Build history of the part. All positions in model axes, mm. A direction names the side the tool comes from. Round coordinates to 2 decimals unless told otherwise and drop trailing zeros. Loops run counter-clockwise (first coordinate to the right, second up) from the corner with the lowest first, then second, coordinate; pieces in that order, holes last. Notation, with made-up numbers: (-37, -23) -> (-14, -23) arc R14 cw to (-14, 3) -> close; hole circle Ø3 at (-30.75, -32.75). An arc over 180 degrees is marked (long way). Put each result on its own line as item: value. Start each with the question number.
Autodesk Fusion 360 part; units mm, degrees
sketch "Sketch1" plane through (0, 0, 0) normal (0, 0, 1) x (1, 0, 0)
  line L0 (-50, 0) -> (-15, 0)
  line L1 (-15, 0) -> (-15, 10)
  line L2 (-15, 10) -> (-50, 10)
  line L3 (-50, 10) -> (-50, 0)
  dimension "d1" = 35
  dimension "d2" = 10
extrude "Extrude1" add sketch "Sketch1" along normal blind 10
sketch "Sketch2" plane through (0, 0, 10) normal (0, 0, 1) x (-1, 0, 0)
  line L0 (50, -10) -> (50, 0)
  line L1 (50, 0) -> (15, 0)
  line L2 (15, 0) -> (15, -10)
  line L3 (15, -10) -> (50, -10)
  line L4 (50, -10) -> (50, -5)
  line L5 (15, -5) -> (15, -10)
  line L6 (15, -5) -> (20, -5)
  line L7 (20, -5) -> (50, -5)
  line L8 (50, -10) -> (15, -10)
extrude "Extrude2" add sketch "Sketch2" along normal blind 25 contours L0 L2 L3 L4 L5 L6 L7 L8
sketch "Sketch3" plane through (0, 5, 0) normal (0, -1, 0) x (1, 0, 0)
  line L0 (-50, 10) -> (-15, 10)
  line L1 (-15, 10) -> (-15, 35)
  line L2 (-15, 35) -> (-50, 35)
  line L3 (-50, 35) -> (-50, 10)
  line L4 (-15, 10) -> (-17, 10)
  line L5 (-17, 10) -> (-17, 12)
  circle A0 centre (-17, 12) radius 1.5
  line L6 (-50, 10) -> (-48, 10)
  circle A1 centre (-48, 12) radius 1.5
  dimension "d7" = 2
  dimension "d8" = 2
  dimension "d9" = 3
  dimension "d10" = 2
  dimension "d11" = 3
extrude "Extrude3" cut sketch "Sketch3" against normal blind 15 contours A0 | A1
sketch "Sketch4" plane through (0, 5, 0) normal (0, -1, 0) x (1, 0, 0)
  circle A0 centre (-17, 12) radius 1.5
  circle A1 centre (-48, 12) radius 1.5
  line L0 (-50, 10) -> (-15, 10)
  line L1 (-15, 10) -> (-15, 35)
  line L2 (-15, 35) -> (-50, 35)
  line L3 (-50, 35) -> (-50, 10)
  line L4 (-17, 10) -> (-17, 25)
  line L5 (-48, 10) -> (-48, 25)
  circle A2 centre (-48, 25) radius 1.5
  circle A3 centre (-17, 25) radius 1.5
  dimension "d14" = 15
  dimension "d15" = 15
  dimension "d16" = 3
  dimension "d17" = 3
extrude "Extrude4" cut sketch "Sketch4" against normal blind 24 contours A2 | A3
sketch "Sketch5" plane through (0, 0, 0) normal (0, 0, -1) x (1, 0, 0)
  line L0 (-50, 0) -> (-50, -10)
  line L1 (-50, -10) -> (-15, -10)
  line L2 (-15, -10) -> (-15, 0)
  line L3 (-15, 0) -> (-50, 0)
sketch "Sketch6" plane through (-50, 0, 0) normal (-1, 0, 0) x (0, -1, 0)
  line L0 (-10, 0) -> (0, 0)
  line L1 (0, 0) -> (0, 10)
  line L2 (0, 10) -> (-5, 10)
  line L3 (-5, 10) -> (-5, 35)
  line L4 (-5, 35) -> (-10, 35)
  line L5 (-10, 35) -> (-10, 0)
  line L6 (0, 10) -> (-10, 10)
  line L7 (-10, 10) -> (-10, 0)
  line L8 (-10, 0) -> (0, 0)
  line L9 (0, 0) -> (0, 10)
extrude "Extrude5" add sketch "Sketch6" along normal blind 3 contours L0 L1 L2 L5 L6 L7 L8 L9
sketch "Sketch7" plane through (-15, 0, 0) normal (1, 0, 0) x (0, 1, 0)
  line L0 (0, 0) -> (10, 0)
  line L1 (10, 0) -> (10, 35)
  line L2 (10, 35) -> (5, 35)
  line L3 (5, 35) -> (5, 10)
  line L4 (5, 10) -> (0, 10)
  line L5 (0, 10) -> (0, 0)
  line L6 (0, 10) -> (10, 10)
  line L7 (10, 10) -> (10, 0)
  line L8 (10, 0) -> (0, 0)
  line L9 (0, 0) -> (0, 10)
extrude "Extrude6" add sketch "Sketch7" along normal blind 3 contours L0 L1 L4 L5 L6 L7 L8 L9
sketch "Sketch8" plane through (0, 0, 0) normal (0, 0, -1) x (1, 0, 0)
sketch "Sketch9" plane through (0, 0, 0) normal (0, 0, -1) x (1, 0, 0)
  line L0 (-53, -10) -> (-52, -10)
  line L1 (-52, -10) -> (-32, -10)
  line L2 (-32, -10) -> (-32, -5)
  line L3 (-32, -5) -> (-15, -5)
  line L4 (-32, -5) -> (-49, -5)
  line L5 (-49, -5) -> (-49, -1)
  line L6 (-49, -5) -> (-49, -9)
  line L7 (-49, -1) -> (-15, -1)
  line L8 (-15, -1) -> (-15, -9)
  line L9 (-15, -9) -> (-49, -9)
  dimension "d24" = 20
  dimension "d25" = 17
  dimension "d26" = 17
  dimension "d27" = 4
  dimension "d28" = 4
extrude "Extrude7" cut sketch "Sketch9" against normal blind 5
Item 1: Cut at D-D on z = 3. Write the cut outline in (x, y).
Item 2: Drop flat-ended pins along their axis: pin 1 (4 mm diameter, centred on y = 8, z = 24, fed in from -X); pin 2 (2.5 mm diameter, centred on x = -33, y = 5.5, fed in from -Z); pin 3 (4 mm diameter, centred on y = 8, z = 21, fed in from +X). Give the stop position or say it passes through.
Item 3: Cut at C-C on y = 8.5. Write the cut outline in (x, z).
Item 4: Cut at B-B on z = 25. Write the cut outline in (x, y), then the cut area to 3 significant figures.
Item 5: Pull direction Z, two halves, no side cores. Call faces 1 (the face through (-49.11, 7.46, 26.01)), 2 (the face through (-49, 5, 2)), 3 (the face through (-32.8, 0.5, 0)): +Z half, -Z half, draft (parallel to the pull), parting line (faces both ways), or undercut.
Item 6: Wall check: line 1 (Z direction, x = -48, y = 6); line 2 (X direction, y = 7, z = 25); line 3 (Y direction, x = -45, z = 3). Give the ranges that are in metal, low to high. Write a range as from..to.
Item 7: 3-axis set-ups, long thin cutter, end or side, ignore diameter. For faces 4 (the face through (-50, 8, 22)), 5 (the face through (-32, 5, 22)), 6 (the face through (-15, 7, 22)), 7 (the face through (-33, 10, 17)), 8 (the face through (-32, 9, 2)): which of +Z, -Z, +X, -X, +Y, -Y reach the whole face in a straight line?
Item 8: Cut at A-A on x = -48. Write the cut outline in (y, z), then the cut area to 3 significant figures.
Ans:
1. outline: (-53, 0) -> (-12, 0) -> (-12, 10) -> (-53, 10) -> close; hole (-49, 1) -> (-15, 1) -> (-15, 9) -> (-49, 9) -> close
2. pin 1: stops at x = -50
2. pin 2: stops at z = 5
2. pin 3: stops at x = -15
3. outline: (-53, 0) -> (-49, 0) -> (-49, 5) -> (-15, 5) -> (-15, 0) -> (-12, 0) -> (-12, 10) -> (-15, 10) -> (-15, 35) -> (-50, 35) -> (-50, 10) -> (-53, 10) -> close; hole circle Ø3 at (-48, 12); hole circle Ø3 at (-48, 25); hole circle Ø3 at (-17, 12); hole circle Ø3 at (-17, 25)
4. outline: (-50, 5) -> (-49.5, 5) -> (-49.5, 10) -> (-50, 10) -> close; (-46.5, 5) -> (-18.5, 5) -> (-18.5, 10) -> (-46.5, 10) -> close; (-15.5, 5) -> (-15, 5) -> (-15, 10) -> (-15.5, 10) -> close
4. area: 145 mm2
5. face 1: undercut
5. face 2: draft
5. face 3: -Z half
6. line 1: z = 5..10.5, 13.5..23.5, 26.5..35
6. line 2: x = -50..-49.5, -46.5..-18.5, -15.5..-15
6. line 3: y = 0..1, 9..10
7. face 4: +Z, -X, +Y, -Y
7. face 5: +Z, +X, -X, -Y
7. face 6: +Z, +X, +Y, -Y
7. face 7: +Z, -Z, +X, -X, +Y
7. face 8: -Z
8. outline: (0, 0) -> (1, 0) -> (1, 5) -> (9, 5) -> (9, 0) -> (10, 0) -> (10, 10.5) -> (5, 10.5) -> (5, 10) -> (0, 10) -> close; (5, 13.5) -> (10, 13.5) -> (10, 23.5) -> (5, 23.5) -> close; (5, 26.5) -> (10, 26.5) -> (10, 35) -> (5, 35) -> close
8. area: 155 mm2
